Geometry: final body of the model. Coordinates: model frame, mm. Coordinates: 2 decimals unless noted, no trailing zeros. Write each loop counter-clockwise with the first axis right and the second up, starting at its lowest first coordinate (ties: lowest second). Pieces come first, ordered by that corner, then holes. Notation, with made-up numbers: M -15,-4.75 L -6,-4.75 A16 cw -6,8.25 Z; hole C 61,36 d5. An arc over 180 degrees is marked long. Write item = value, one per line. Start each with the question number.
Item 1: Section B-B on x = 19.5. Output: boundary loops of the cut face in (y, z).
Item 2: Ray query, L1, parallel to X at y = 0.2, z = -23; L2, parallel to Z at x = 11.5, y = 1.5; L3, parallel to Z at x = 11, y = 1.45. Return the intervals inside material, ascending. Write a range as [from, to].
Item 3: Section C-C on y = 1.2. Give the number of separate pieces and of enclosed holes in the cut face, plus the area to 3 significant figures.
Item 4: First-contact query: pin 1 Ø1 at (x, y) = (62.5, 1) entering from -Z; pin 2 Ø2 at (x, z) = (105.59, -47.97) entering from -Y; pin 3 Ø1 at (y, z) = (1.5, -25.5) entering from +X. Flat tips, straight axial feed; report the tip coordinate or a pass-through.
Item 5: Section A-A on x = 105.5. Output: boundary loops of the cut face in (y, z), plus the area to 3 significant figures.
Item 6: Section D-D on x = 64.5. Output: boundary loops of the cut face in (y, z), plus the area to 3 significant figures.
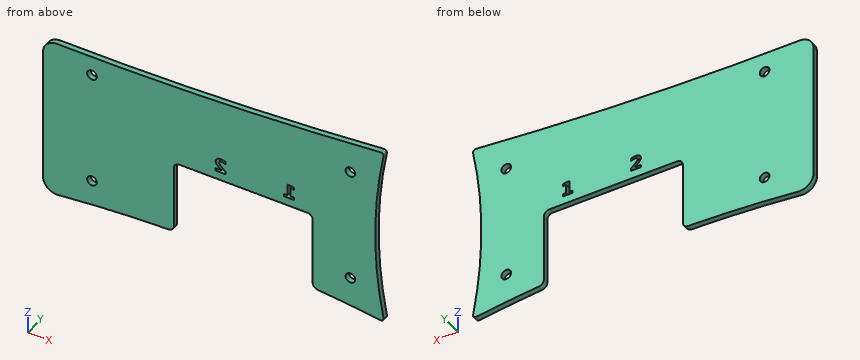
from build123d import *

# Parameters (mm, degrees)
CROQUIS1_R              = 2.175
SALIENTE_EXTRUIR1_DEPTH = 2
CROQUIS2_R              = 2.175
CROQUIS2_R_2            = 1.75
SALIENTE_EXTRUIR2_DEPTH = 2
CROQUIS3_W              = 50
CROQUIS3_H              = 30
CORTAR_EXTRUIR1_DEPTH   = 2
REDONDEO1_R             = 2
CORTAR_EXTRUIR2_DEPTH   = 2


with BuildPart() as part:
    # Croquis1 → Saliente-Extruir1 (new body)
    with BuildSketch(Plane(origin=(0, 0, 0), x_dir=(1, 0, 0), z_dir=(0, 1, 0))):
        with BuildLine():
            Line((-5.038018703, 53.362868047), (-5.038018703, 4.999855456))
            ThreePointArc((-5.038018703, 4.999855456), (-3.560085318, 1.450905363), (0, 0))
            ThreePointArc((0, 0), (58.295330849, -1.055734), (116.459334215, -5.106522257))
            ThreePointArc((116.459334215, -5.106522257), (117.294081225, -4.78404952), (117.536525368, -3.922648293))
            ThreePointArc((117.536525368, -3.922648293), (114.552978917, 27.433067341), (117.524427855, 58.789931717))
            ThreePointArc((117.524427855, 58.789931717), (117.266809662, 59.667185903), (116.403513339, 59.968286381))
            ThreePointArc((116.403513339, 59.968286381), (58.510820536, 55.521592761), (0.515666266, 58.332116778))
            ThreePointArc((0.515666266, 58.332116778), (-3.372053433, 57.089020542), (-5.038018703, 53.362868047))
        make_face()
        with Locations((105.593713907, 6.96520452)):
            Circle(CROQUIS1_R, mode=Mode.SUBTRACT)
        with Locations((105.593713907, 47.96520452)):
            Circle(CROQUIS1_R, mode=Mode.SUBTRACT)
        with Locations((12.593713907, 47.96520452)):
            Circle(CROQUIS1_R, mode=Mode.SUBTRACT)
        with Locations((12.593713907, 6.96520452)):
            Circle(CROQUIS1_R, mode=Mode.SUBTRACT)
    extrude(amount=SALIENTE_EXTRUIR1_DEPTH)

    # Croquis2 → Saliente-Extruir2 (add)
    with BuildSketch(Plane(origin=(0, 2, 0), x_dir=(1, 0, 0), z_dir=(0, 1, 0))):
        with Locations((12.593713907, 6.96520452)):
            Circle(CROQUIS2_R)
        with Locations((12.593713907, 6.96520452)):
            Circle(CROQUIS2_R_2, mode=Mode.SUBTRACT)
        with Locations((105.593713907, 6.96520452)):
            Circle(CROQUIS2_R)
        with Locations((105.593713907, 6.96520452)):
            Circle(CROQUIS2_R_2, mode=Mode.SUBTRACT)
        with Locations((105.593713907, 47.96520452)):
            Circle(CROQUIS2_R)
        with Locations((105.593713907, 47.96520452)):
            Circle(CROQUIS2_R_2, mode=Mode.SUBTRACT)
        with Locations((12.593713907, 47.96520452)):
            Circle(CROQUIS2_R)
        with Locations((12.593713907, 47.96520452)):
            Circle(CROQUIS2_R_2, mode=Mode.SUBTRACT)
    extrude(amount=-SALIENTE_EXTRUIR2_DEPTH)

    # Croquis3 → Cortar-Extruir1 (cut)
    with BuildSketch(Plane.XZ):
        with Locations((67.042264057, -43.977959042)):
            Rectangle(CROQUIS3_W, CROQUIS3_H)
    extrude(amount=-CORTAR_EXTRUIR1_DEPTH, mode=Mode.SUBTRACT)

    # Redondeo1
    redondeo1_edges = [part.edges().sort_by_distance(p)[0] for p in [
        (92.042264057, 1, -57.208472181),
        (42.042264057, 1, -55.581052497),
        (92.042264057, 1, -28.977959042),
        (42.042264057, 1, -28.977959042),
    ]]
    fillet(redondeo1_edges, radius=REDONDEO1_R)

    # Croquis5 → Cortar-Extruir2 (cut)
    with BuildSketch(Plane.XZ):
        Polygon((85.245219848, -25.091883093), (84.105979342, -25.091883093), (84.105979342, -21.864034991), (85.245219848, -22.117199548), (85.245219848, -21.231123599), (84.105979342, -20.977959042), (82.903447696, -20.977959042), (82.903447696, -25.091883093), (81.76420719, -25.091883093), (81.76420719, -25.977959042), (85.245219848, -25.977959042), align=None)
        with BuildLine():
            Line((59.23923156, -25.028591953), (57.043820167, -25.028591953))
            Line((57.043820167, -25.028591953), (57.043820167, -25.977959042))
            Line((57.043820167, -25.977959042), (60.651415104, -25.977959042))
            Line((60.651415104, -25.977959042), (60.651415104, -25.028591953))
            Line((60.651415104, -25.028591953), (58.849595484, -23.39686727))
            add(Edge.make_bspline(
                [(58.849595484, -23.39686727), (58.811179508, -23.360453729), (58.737347895, -23.290470593), (58.638846251, -23.181308349), (58.556039894, -23.073418427), (58.488647556, -22.9656663), (58.436579253, -22.857270202), (58.399356742, -22.7471273), (58.376788079, -22.635006299), (58.374215363, -22.559348688), (58.372934091, -22.521669485)],
                knots=[0, 0, 0, 0, 0.000158749, 0.0003051, 0.000440586, 0.000566273, 0.000685704, 0.000800474, 0.000914321, 0.001027271, 0.001027271, 0.001027271, 0.001027271], degree=3))
            add(Edge.make_bspline(
                [(58.372934091, -22.521669485), (58.373734222, -22.492954485), (58.375303557, -22.436634341), (58.386395262, -22.354534572), (58.403952327, -22.27651726), (58.429843029, -22.202852998), (58.463496065, -22.13358734), (58.504554072, -22.068788136), (58.55230711, -22.007870779), (58.607454048, -21.95191928), (58.668588665, -21.901761082), (58.734750953, -21.857510772), (58.805768742, -21.820347701), (58.881617778, -21.78880132), (58.962945343, -21.766978108), (59.048496141, -21.750115414), (59.138706913, -21.738517651), (59.200626269, -21.737813177), (59.232309091, -21.737452713)],
                knots=[0, 0, 0, 0, 8.6127e-05, 0.000168926, 0.000248089, 0.000325655, 0.000402613, 0.000478613, 0.000555374, 0.000634395, 0.000713787, 0.00079223, 0.000872741, 0.000953911, 0.001038132, 0.001124825, 0.001215473, 0.001310456, 0.001310456, 0.001310456, 0.001310456], degree=3))
            add(Edge.make_bspline(
                [(59.232309091, -21.737452713), (59.283483298, -21.739078861), (59.388654688, -21.742420863), (59.549919694, -21.767428422), (59.717848281, -21.808754845), (59.893140764, -21.864093074), (60.074545452, -21.936143809), (60.262356788, -22.023375721), (60.45625408, -22.126411077), (60.585178282, -22.203946693), (60.651415104, -22.243781827)],
                knots=[0, 0, 0, 0, 0.000153487, 0.000315441, 0.000488379, 0.00067197, 0.000866447, 0.001073517, 0.001292942, 0.001524792, 0.001524792, 0.001524792, 0.001524792], degree=3))
            Line((60.651415104, -22.243781827), (60.651415104, -21.16783246))
            add(Edge.make_bspline(
                [(60.651415104, -21.16783246), (60.580024738, -21.143346845), (60.438298447, -21.094737271), (60.22526093, -21.029932245), (60.012697372, -20.977227076), (59.802522423, -20.931042179), (59.593297587, -20.895451623), (59.386119489, -20.869557673), (59.180786794, -20.854336471), (59.044767338, -20.852359369), (58.977166686, -20.851376764)],
                knots=[0, 0, 0, 0, 0.000226414, 0.000449484, 0.000667747, 0.000883244, 0.001094922, 0.001304182, 0.001509426, 0.001712216, 0.001712216, 0.001712216, 0.001712216], degree=3))
            add(Edge.make_bspline(
                [(58.977166686, -20.851376764), (58.905262711, -20.85238657), (58.765150213, -20.854354283), (58.561236326, -20.873331522), (58.369861257, -20.904710686), (58.190983935, -20.948290574), (58.02362641, -21.003040105), (57.869196403, -21.072605629), (57.726828905, -21.153727261), (57.597883717, -21.246919107), (57.482225307, -21.350888685), (57.382280492, -21.4662574), (57.296169552, -21.590505745), (57.226253234, -21.725372616), (57.173379692, -21.870513757), (57.134463349, -22.024856787), (57.111652808, -22.189040836), (57.108650287, -22.301727129), (57.107111307, -22.359485941)],
                knots=[0, 0, 0, 0, 0.000215667, 0.00042025, 0.000613718, 0.000796966, 0.000972092, 0.001141183, 0.0013042, 0.001462847, 0.001617578, 0.001769683, 0.001919729, 0.002070114, 0.002224056, 0.002382117, 0.002546867, 0.00272011, 0.00272011, 0.00272011, 0.00272011], degree=3))
            add(Edge.make_bspline(
                [(57.107111307, -22.359485941), (57.109580941, -22.426905794), (57.114488685, -22.560884856), (57.153988801, -22.758138197), (57.220643738, -22.947717445), (57.29612885, -23.101195245), (57.373494642, -23.224613477), (57.44767263, -23.324133234), (57.534574057, -23.431842783), (57.636091495, -23.546775274), (57.751967056, -23.669028973), (57.881725831, -23.799417167), (58.024876774, -23.938220802), (58.127076255, -24.031061987), (58.180093902, -24.079224865)],
                knots=[0, 0, 0, 0, 0.00020215, 0.000401719, 0.000600628, 0.000803627, 0.00091338, 0.001037201, 0.001175739, 0.001328495, 0.001497091, 0.001681002, 0.001880326, 0.002095195, 0.002095195, 0.002095195, 0.002095195], degree=3))
            Line((58.180093902, -24.079224865), (59.23923156, -25.028591953))
        make_face()
    extrude(amount=-CORTAR_EXTRUIR2_DEPTH, mode=Mode.SUBTRACT)


solid = part.part
Responses:
q1.outline = M 0,-56.61 L 2,-56.61 L 2,0.02 L 0,0.02 Z
q2.L1 = [-5.04, 57.25], [58.51, 82.9], [84.11, 114.61]
q2.L2 = [-57.24, -49.33], [-46.6, -8.33], [-5.6, -0.03]
q2.L3 = [-57.28, -48.69], [-47.24, -7.69], [-6.24, -0.03]
q3.separate_pieces = 1
q3.enclosed_holes = 6
q3.area = 5,610 mm²
q4.pin_1 = -28.98
q4.pin_2 = through
q4.pin_3 = 114.57
q5.outline = M 0,-58.57 L 2,-58.57 L 2,-49.71 L 0,-49.71 Z; M 0,-46.22 L 2,-46.22 L 2,-8.71 L 0,-8.71 Z; M 0,-5.22 L 2,-5.22 L 2,4.11 L 0,4.11 Z
q5.area = 111 mm²
q6.outline = M 0,-28.98 L 2,-28.98 L 2,1.34 L 0,1.34 Z
q6.area = 60.6 mm²
